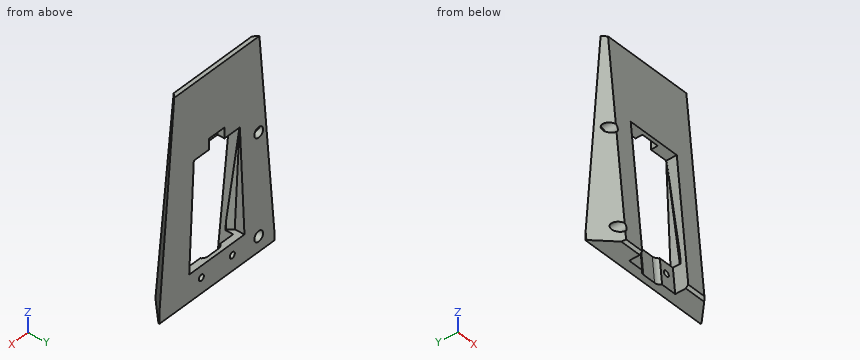
```python
from build123d import *
from OCP.BRepFilletAPI import BRepFilletAPI_MakeChamfer

# Parameters (mm, degrees)
BOSS_EXTRUDE1_START = 126.292269218
BOSS_EXTRUDE1_DEPTH = 75
CHAMFER1_SIZE       = 12
CHAMFER2_SIZE       = 1.5
CHAMFER2_SIZE2      = 1.38459352
CUT_EXTRUDE1_REACH  = 228.979
SKETCH5_R           = 2.875
CUT_EXTRUDE2_DEPTH  = 227.978701072
SKETCH6_W           = 30
SKETCH6_H           = 15
SKETCH6_R           = 2.875
SKETCH6_H_2         = 60
CUT_EXTRUDE3_DEPTH  = 227.978701072
BOSS_EXTRUDE2_START = 148.792269218
BOSS_EXTRUDE2_DEPTH = 30
CUT_EXTRUDE4_DEPTH  = 30
SKETCH11_R          = 1.65
CUT_EXTRUDE5_DEPTH  = 227.978701072
SKETCH12_W          = 10
SKETCH12_H          = 3.906967626
CUT_EXTRUDE6_DEPTH  = 6
CHAMFER3_SIZE       = 2.7
CHAMFER3_SIZE2      = 2.711828512


# Read off the part's stored shape, not the designer's step: Boss-Extrude1, Boss-Extrude2
with BuildPart() as part:
    # Boss-Extrude1 outline → Boss-Extrude1 (new body)
    with BuildSketch(Plane.YZ.offset(BOSS_EXTRUDE1_START)):
        Polygon((-26.968617391, -104.155083501), (-14.5, -104.155083501), (-14.5, 12.696761663), (-16.745405627, 12.696761663), align=None)
    extrude(amount=BOSS_EXTRUDE1_DEPTH)

    # Chamfer1
    chamfer1_edges = [part.edges().sort_by_distance(p)[0] for p in [
        (201.292269218, -21.857011509, -45.729160919),
        (126.292269218, -21.857011509, -45.729160919),
    ]]
    chamfer(chamfer1_edges, length=CHAMFER1_SIZE)

    # Chamfer2
    chamfer2_edges = [part.edges().sort_by_distance(p)[0] for p in [
        (163.792269218, -26.968617391, -104.155083501),
    ]]
    chamfer2_side = [part.faces().sort_by_distance(p)[0] for p in [
        (163.792269218, -20.328588559, -104.155083501),
    ]]
    chamfer(chamfer2_edges, length=CHAMFER2_SIZE, length2=CHAMFER2_SIZE2, reference=chamfer2_side[0])

    # Cut-Extrude1: up to this plane
    cut_extrude1_end = Plane(origin=(0, -14.732006126, 1.288883527), z_dir=(0, -0.9961946980917461, 0.08715574274765119))
    # Sketch3 → Cut-Extrude1 (cut, up to the surface)
    with BuildSketch(Plane(origin=(0, -14.5, 0), x_dir=(1, 0, 0), z_dir=(0, 1, 0)), mode=Mode.PRIVATE) as cut_extrude1_sk1:
        Polygon((145.792269218, 89.155083501), (181.792269218, 89.155083501), (178.792269218, 29.155083501), (148.792269218, 29.155083501), align=None)
    cut_extrude1_tool1 = split(extrude(cut_extrude1_sk1.sketch, amount=-CUT_EXTRUDE1_REACH, mode=Mode.PRIVATE), bisect_by=cut_extrude1_end, keep=Keep.BOTH, mode=Mode.PRIVATE)
    add(cut_extrude1_tool1.solids().sort_by_distance((163.792269, -14.5, -60.064174))[0], mode=Mode.SUBTRACT)

    # Sketch5 → Cut-Extrude2 (cut, through all)
    with BuildSketch(Plane(origin=(0, -14.5, 0), x_dir=(1, 0, 0), z_dir=(0, 1, 0))):
        with Locations(Location((173.869198237, 95.613531365, 0), (0, 0, 270))):
            Circle(SKETCH5_R)
        with Locations(Location((136.518193504, 95.738532693, 0), (0, 0, 270))):
            Circle(SKETCH5_R)
        with Locations(Location((136.518193504, 39.320563904, 0), (0, 0, 270))):
            Circle(SKETCH5_R)
    extrude(amount=-CUT_EXTRUDE2_DEPTH, mode=Mode.SUBTRACT)

    # Sketch6 → Cut-Extrude3 (cut, through all)
    # profile 1 of 2: a face of its own
    with BuildSketch(Plane(origin=(0, -14.5, 0), x_dir=(1, 0, 0), z_dir=(0, 1, 0))):
        with Locations((163.792269218, 96.655083501)):
            Rectangle(SKETCH6_W, SKETCH6_H)
        with Locations((173.869198237, 95.613531365)):
            Circle(SKETCH6_R, mode=Mode.SUBTRACT)
    # profile 2 of 2: a face of its own
    with BuildSketch(Plane(origin=(0, -14.5, 0), x_dir=(1, 0, 0), z_dir=(0, 1, 0))):
        with Locations((163.792269218, 59.155083501)):
            Rectangle(SKETCH6_W, SKETCH6_H_2)
    extrude(amount=-CUT_EXTRUDE3_DEPTH, mode=Mode.SUBTRACT)

    # Boss-Extrude2 outline → Boss-Extrude2 (add)
    with BuildSketch(Plane.YZ.offset(BOSS_EXTRUDE2_START)):
        Polygon((-19.540350593, -104.155083501), (-14.5, -104.155083501), (-14.5, -89.155083501), (-18.22802064, -89.155083501), align=None)
    extrude(amount=BOSS_EXTRUDE2_DEPTH)

    # Sketch9 → Cut-Extrude4 (cut)
    with BuildSketch(Plane(origin=(0, -9.191601139, -105.06048176), x_dir=(-1, 0, 0), z_dir=(0, -0.08715574274765119, -0.9961946980917462))):
        with BuildLine():
            Line((-167.292269218, -8.738279996), (-160.292269218, -8.738279996))
            ThreePointArc((-160.292269218, -8.738279996), (-156.792269218, -12.238279996), (-160.292269218, -15.738279996))
            Line((-160.292269218, -15.738279996), (-167.292269218, -15.738279996))
            ThreePointArc((-167.292269218, -15.738279996), (-170.792269218, -12.238279996), (-167.292269218, -8.738279996))
        make_face()
    extrude(amount=-CUT_EXTRUDE4_DEPTH, mode=Mode.SUBTRACT)

    # Sketch11 → Cut-Extrude5 (cut, through all)
    with BuildSketch(Plane(origin=(0, -14.5, 0), x_dir=(1, 0, 0), z_dir=(0, 1, 0))):
        with Locations(Location((173.869198237, 95.613531365, 0), (0, 0, 270))):
            Circle(SKETCH11_R)
        with Locations(Location((153.7153402, 95.613531365, 0), (0, 0, 270))):
            Circle(SKETCH11_R)
    extrude(amount=-CUT_EXTRUDE5_DEPTH, mode=Mode.SUBTRACT)

    # Sketch12 → Cut-Extrude6 (cut)
    with BuildSketch(Plane(origin=(0, 0, -29.155083501), x_dir=(-1, 0, 0), z_dir=(0, 0, -1))):
        with Locations((-163.792269218, -16.453483813)):
            Rectangle(SKETCH12_W, SKETCH12_H)
    extrude(amount=-CUT_EXTRUDE6_DEPTH, mode=Mode.SUBTRACT)

    # Chamfer3: one chamfer whose edges measure the first distance from different faces: ONE call of the kernel's chamfer builder (chamfer() names one face for all edges)
    chamfer3_edges_1 = [part.edges().sort_by_distance(p)[0] for p in [
        (180.292269218, -20.020168019, -59.155083501),
    ]]
    chamfer3_side_1 = [part.faces().sort_by_distance(p)[0] for p in [
        (180.530002915, -17.468074044, -63.909757447),
    ]]
    chamfer3_edges_2 = [part.edges().sort_by_distance(p)[0] for p in [
        (147.292269218, -20.020168019, -59.155083501),
    ]]
    chamfer3_side_2 = [part.faces().sort_by_distance(p)[0] for p in [
        (147.054535521, -17.468074044, -63.909757447),
    ]]
    chamfer3 = BRepFilletAPI_MakeChamfer(part.part.solid().wrapped)
    for e in chamfer3_edges_1:
        chamfer3.Add(CHAMFER3_SIZE, CHAMFER3_SIZE2, e.wrapped, chamfer3_side_1[0].wrapped)  # the first distance lies on this face
    for e in chamfer3_edges_2:
        chamfer3.Add(CHAMFER3_SIZE, CHAMFER3_SIZE2, e.wrapped, chamfer3_side_2[0].wrapped)  # the first distance lies on this face
    add(Compound.cast(chamfer3.Shape()), mode=Mode.REPLACE)


solid = part.part
```
Part model, mm, in its own coordinate system. Round coordinates to 2 decimals unless told otherwise and drop trailing zeros. Write each loop counter-clockwise with the first axis right and the second up, starting at its lowest first coordinate (ties: lowest second). Pieces come first, ordered by that corner, then holes. Notation, with made-up numbers: (41.5, 56) -> (98.5, 56) arc R21 ccw to (98.5, 64) -> close; hole circle Ø4 at (24.5, 6). An arc over 180 degrees is marked (long way). Return JSON: item names as keys, results as strings. Group by question number.
Q1. Saw through at D-D on z = -85. Write the cut outline in (x, y).
Q2. Saw through at A-A on x = 164.5. Write the cut outline in (y, z).
Q3. Saw through at C-C on x = 177. Write the cut outline in (y, z).
Q4. Probe L1, parallel to Z at x = 160, y = -16; L2, parallel to X at y = -17, z = -33; L3, parallel to X at y = -16.75, z = -43.5. List the from-to ranges inside material, lowest first. Write a range as [from, to].
Q5. Saw through at B-B on z = -53. Write the cut outline in (x, y), plus the area to 3 significant figures.
Q6. Pin check, flat tips, straight feed: pin 1 (1 mm diameter, centred on x = 185, z = -43.5, fed in from -Y); pin 2 (4 mm diameter, centred on y = -22, z = -56.5, fed in from -X); pin 3 (2 mm diameter, centred on x = 153.72, z = -95.61, fed in from +Y); pin 4 (1 mm diameter, centred on x = 138.5, z = -57, fed in from -Y). Stop position of each tip, or through.
Answer:
{
 "1": {"outline": "(127.54, -14.5) -> (138.29, -25.29) -> (148.79, -25.29) -> (148.79, -22.28) -> (148.72, -22.28) -> (146, -19.57) -> (146, -14.5) -> close; (178.79, -25.29) -> (189.29, -25.29) -> (200.04, -14.5) -> (181.58, -14.5) -> (181.58, -19.57) -> (178.87, -22.28) -> (178.79, -22.28) -> close"},
 "2": {"outline": "(-20.41, -29.16) -> (-18.41, -29.16) -> (-18.41, -23.16) -> (-14.5, -23.16) -> (-14.5, 12.7) -> (-16.75, 12.7) -> close; (-17.88, -104.16) -> (-14.5, -104.16) -> (-14.5, -89.16) -> (-16.57, -89.16) -> close"},
 "3": {"outline": "(-20.41, -29.16) -> (-14.5, -29.16) -> (-14.5, 12.7) -> (-16.75, 12.7) -> close; (-19.54, -104.16) -> (-14.5, -104.16) -> (-14.5, -89.16) -> (-18.23, -89.16) -> close"},
 "4": {"L1": "[-104.16, -89.16], [-23.16, 12.7]", "L2": "[134.56, 148.79], [178.79, 193.02]", "L3": "[133.4, 148.79], [178.79, 194.19]"},
 "5": {"outline": "(130.33, -14.5) -> (138.29, -22.49) -> (148.79, -22.49) -> (148.79, -17.96) -> (147.6, -16.77) -> (147.6, -14.5) -> close; (178.79, -22.49) -> (189.29, -22.49) -> (197.25, -14.5) -> (179.98, -14.5) -> (179.98, -16.77) -> (178.79, -17.96) -> close", "area": "225 mm2"},
 "6": {"pin 1": "y = -21.71", "pin 2": "x = 135.5", "pin 3": "through", "pin 4": "y = -22.89"}
}
